Verification items for the finished model (mm, model axes). Coordinates: 2 decimals unless noted, no trailing zeros. Loops run counter-clockwise (first coordinate to the right, second up) from the corner with the lowest first, then second, coordinate; pieces in that order, holes last. Notation, with made-up numbers: (73, 68) - (91, 68) arc R25 cw to (91, 84) - close; hole circle Ø5 at (44.5, 70). An arc over 180 degrees is marked (long way). One line per item, written item: value. Start each with the question number.
(1) Section check B-B (x = 0). Record the boundary of the cut face in (y, z) (3 decimals), plus the area to 3 significant figures.
(2) Gauge pin test, flat ends, axial feed: P1, Ø1, axis at x = -34, z = 55.5, coming from the -Y side; P2, Ø1, axis at x = -152, y = 4, coming from the +Z side. Record the tip position at first contact, or that the pin passes through.
(3) Section check C-C (y = 4.25). Record the boundary of the cut face in (x, z) (3 decimals), plus the area to 3 significant figures.
(4) Section check A-A (z = 63.5). Record the boundary of the cut face in (x, y).
(5) Thickness scan on probe 1 along Z at (x, y) = (0, 0.65) (3 decimals); probe 2 along X at (y, z) = (4.25, 63.5); probe 3 along X at (y, z) = (1.5, -7) (3 decimals). Record the ranges inside material, lowest first. Write a range as [from, to].
(6) Section check D-D (x = 109.5). Record the boundary of the cut face in (y, z).
Autodesk Inventor part; units mm, degrees
ref_plane "YZ Plane" through (0, 0, 0) normal (1, 0, 0) x (0, 1, 0)
ref_plane "XZ Plane" through (0, 0, 0) normal (0, 1, 0) x (-1, 0, 0)
ref_plane "XY Plane" through (0, 0, 0) normal (0, 0, 1) x (1, 0, 0)
sketch "Sketch1" plane through (0, 0, 0) normal (0, 1, 0) x (-1, 0, 0)
  line L0 (-203.2, 84.1682) -> (-84.1682, 203.2)
  line L1 (-84.1682, 203.2) -> (84.1682, 203.2)
  line L2 (84.1682, 203.2) -> (203.2, 84.1682)
  line L3 (203.2, 84.1682) -> (203.2, -84.1682)
  line L4 (203.2, -84.1682) -> (84.1682, -203.2)
  line L5 (84.1682, -203.2) -> (-84.1682, -203.2)
  line L6 (-84.1682, -203.2) -> (-203.2, -84.1682)
  line L7 (-203.2, -84.1682) -> (-203.2, 84.1682)
  point P0 (0, 0)
  point P1 (0, 0)
  dimension "d0" = 406.4
extrude "Extrusion1" add sketch "Sketch1" along normal blind 5.5563
sketch "Sketch2" plane through (0, 5.5563, 0) normal (0, 1, 0) x (1, 0, 0)
  line L0 (9.525, -9.525) -> (-9.525, -9.525)
  line L1 (-9.525, -9.525) -> (-9.525, 9.525)
  line L2 (-9.525, 9.525) -> (9.525, 9.525)
  line L3 (9.525, 9.525) -> (9.525, -9.525)
  circle A0 centre (0, -63.5) radius 12.7
  point P0 (0, 0)
  dimension "d3" = 19.05
  dimension "d4" = 19.05
  dimension "d5" = 9.525
  dimension "d6" = 9.525
  dimension "d9" = 25.4
  dimension "d10" = 63.5
extrude "Extrusion2" cut sketch "Sketch2" against normal through all
equation "\"d0\" = BaseWidth"
equation "\"d3\" = MastWidth"
equation "\"d4\" = d3"
equation "\"d9\" = WireHoleDiameter"
properties part number "Robot-Upper-Base" material "Wood (Birch)"
Responses:
1. outline: (0, -203.2) - (5.556, -203.2) - (5.556, -9.525) - (0, -9.525) - close; (0, 9.525) - (5.556, 9.525) - (5.556, 50.8) - (0, 50.8) - close; (0, 76.2) - (5.556, 76.2) - (5.556, 203.2) - (0, 203.2) - close
1. area: 2,010 mm²
2. P1: stops at y = 0
2. P2: stops at z = 135.87
3. outline: (-203.2, -84.168) - (-84.168, -203.2) - (84.168, -203.2) - (203.2, -84.168) - (203.2, 84.168) - (84.168, 203.2) - (-84.168, 203.2) - (-203.2, 84.168) - close; hole circle Ø25.4 at (0, 63.5); hole (-9.525, -9.525) - (9.525, -9.525) - (9.525, 9.525) - (-9.525, 9.525) - close
3. area: 136,000 mm²
4. outline: (-203.2, 0) - (-12.7, 0) - (-12.7, 5.56) - (-203.2, 5.56) - close; (12.7, 0) - (203.2, 0) - (203.2, 5.56) - (12.7, 5.56) - close
5. probe 1: z = [-203.2, -9.525], [9.525, 50.8], [76.2, 203.2]
5. probe 2: x = [-203.2, -12.7], [12.7, 203.2]
5. probe 3: x = [-203.2, -9.525], [9.525, 203.2]
6. outline: (0, -177.87) - (5.56, -177.87) - (5.56, 177.87) - (0, 177.87) - close
